Could you check a few things on this model? Use its own coordinates, in mm. Give positions to 0.01 mm unless a question says otherwise; leave off trailing zeros. Order: outer loops, then holes, each group sorted by start corner. A loop starts at its lowest first (then second) coordinate and runs counter-clockwise, first axis right, second up.
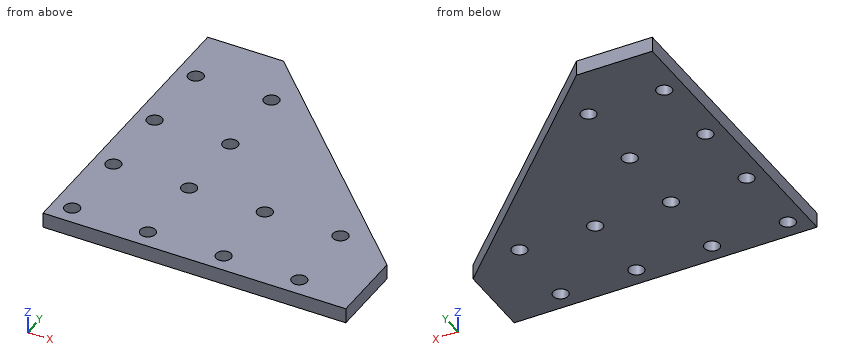
from build123d import *

# Parameters (mm, degrees)
SKETCH1_R           = 4
BOSS_EXTRUDE1_DEPTH = 8


with BuildPart() as part:
    # Sketch1 → Boss-Extrude1 (new body)
    with BuildSketch(Plane.XY):
        Polygon((0, 0), (0, 160), (40, 160), (160, 40), (160, 0), align=None)
        with Locations((10, 10)):
            Circle(SKETCH1_R, mode=Mode.SUBTRACT)
        with Locations((50, 10)):
            Circle(SKETCH1_R, mode=Mode.SUBTRACT)
        with Locations((90, 10)):
            Circle(SKETCH1_R, mode=Mode.SUBTRACT)
        with Locations((10, 90)):
            Circle(SKETCH1_R, mode=Mode.SUBTRACT)
        with Locations((10, 50)):
            Circle(SKETCH1_R, mode=Mode.SUBTRACT)
        with Locations((130, 10)):
            Circle(SKETCH1_R, mode=Mode.SUBTRACT)
        with Locations((10, 130)):
            Circle(SKETCH1_R, mode=Mode.SUBTRACT)
        with Locations((130, 50)):
            Circle(SKETCH1_R, mode=Mode.SUBTRACT)
        with Locations((90, 50)):
            Circle(SKETCH1_R, mode=Mode.SUBTRACT)
        with Locations((50, 50)):
            Circle(SKETCH1_R, mode=Mode.SUBTRACT)
        with Locations((50, 130)):
            Circle(SKETCH1_R, mode=Mode.SUBTRACT)
        with Locations((50, 90)):
            Circle(SKETCH1_R, mode=Mode.SUBTRACT)
    extrude(amount=BOSS_EXTRUDE1_DEPTH)


solid = part.part
Item 1: Imagine slicing it at D-D on y = 130. List the corners of the cut face in (x, z) for me.
Findings:
outline: (0, 0) - (6, 0) - (6, 8) - (0, 8) - close; (14, 0) - (46, 0) - (46, 8) - (14, 8) - close; (54, 0) - (70, 0) - (70, 8) - (54, 8) - close
Item 2: For pin 1 (6.5 mm diameter, centred on x = 130, y = 10, fed in from -Z); pin 2 (3 mm diameter, centred on x = 68, z = 5.5, fed in from +Y); pin 3 (3 mm diameter, centred on x = 140, z = 4.5, fed in from +Y); pin 4 (1.5 mm diameter, centred on y = 82, z = 7, fed in from +X), each with a flat end and sliding along its axis, tell me the tip position at first contact or that it passes through.
Findings:
pin 1: passes through
pin 2: stops at y = 133.5
pin 3: stops at y = 61.5
pin 4: stops at x = 118.75
Item 3: Imagine slicing it at C-C on x = 10. List the corners of the cut face in (y, z) for me, then the cut area to 3 significant figures.
Findings:
outline: (0, 0) - (6, 0) - (6, 8) - (0, 8) - close; (14, 0) - (46, 0) - (46, 8) - (14, 8) - close; (54, 0) - (86, 0) - (86, 8) - (54, 8) - close; (94, 0) - (126, 0) - (126, 8) - (94, 8) - close; (134, 0) - (160, 0) - (160, 8) - (134, 8) - close
area: 1,020 mm2
Item 4: Imagine slicing it at A-A on y = 50. List the corners of the cut face in (x, z) for me, then the cut area to 3 significant figures.
Findings:
outline: (0, 0) - (6, 0) - (6, 8) - (0, 8) - close; (14, 0) - (46, 0) - (46, 8) - (14, 8) - close; (54, 0) - (86, 0) - (86, 8) - (54, 8) - close; (94, 0) - (126, 0) - (126, 8) - (94, 8) - close; (134, 0) - (150, 0) - (150, 8) - (134, 8) - close
area: 944 mm2
Item 5: Please list where these lines run through material, in increasing order: line 1 along X through (y, z) = (8.5, 4.25); line 2 along Y through (x, z) = (12.5, 4.5); line 3 along X through (y, z) = (52, 2.25).
Findings:
line 1: x = 0 to 6.29, 13.71 to 46.29, 53.71 to 86.29, 93.71 to 126.29, 133.71 to 160
line 2: y = 0 to 6.88, 13.12 to 46.88, 53.12 to 86.88, 93.12 to 126.88, 133.12 to 160
line 3: x = 0 to 6.54, 13.46 to 46.54, 53.46 to 86.54, 93.46 to 126.54, 133.46 to 148
Item 6: Imagine slicing it at B-B on z = 5. Give the number of separate pieces and of enclosed holes in the cut face, then the cut area to 3 significant figures.
Findings:
separate pieces: 1
enclosed holes: 12
area: 17,800 mm2
